Here's how the part is built. I have some questions about the finished solid (model axes, mm). Face numbers are marked on the shaded views. A direction names the side the tool comes from. Coordinates: 2 decimals unless noted, no trailing zeros. Loops run counter-clockwise (first coordinate to the right, second up) from the corner with the lowest first, then second, coordinate; pieces in that order, holes last.
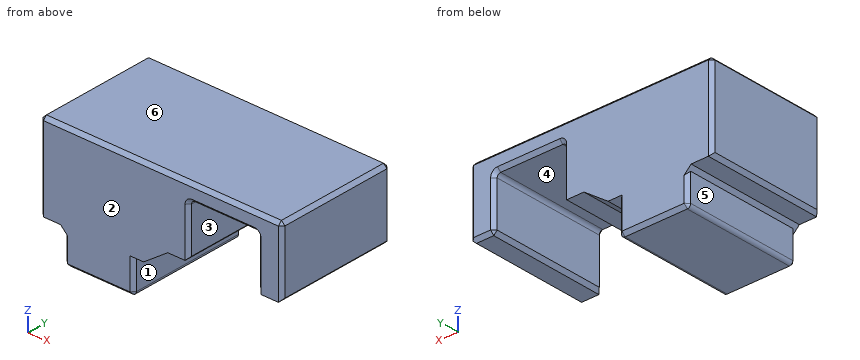
```python
from build123d import *

# Parameters (mm, degrees)
F1_DEPTH = 17.5
F2_SIZE  = 1
F3_R     = 1
F4_SIZE  = 1


with BuildPart() as f1:
    # F0 (on Front) → F1 (new body, symmetric)
    with BuildSketch(Plane.XZ):
        Polygon((33.969838, 0), (40.969838, 0), (40.969838, 20), (-29.030162, 20), (-29.030162, -5), (-22.030162, -5), (-22.030162, -15), (-2.030162, -15), (-2.030162, -5), (0.98608, -5), (7.969838, 0), (13.969838, 0), (13.969838, 15), (33.969838, 15), align=None)
    extrude(amount=F1_DEPTH, both=True)

    # F2
    f2_edges = [f1.edges().sort_by_distance(p)[0] for p in [
        (40.969838, 0, 0),
        (40.969838, -17.5, 10),
        (40.969838, 0, 20),
        (40.969838, 17.5, 10),
        (5.969838, -17.5, 20),
        (5.969838, 17.5, 20),
        (-29.030162, 0, 20),
        (-29.030162, -17.5, 7.5),
        (-29.030162, 17.5, 7.5),
        (-29.030162, 0, -5),
        (-22.030162, 0, -5),
    ]]
    chamfer(f2_edges, length=F2_SIZE)

    # F3
    f3_edges = [f1.edges().sort_by_distance(p)[0] for p in [
        (-22.030162, 0, -15),
        (-2.030162, 0, -15),
        (13.969838, 0, 15),
        (33.969838, 0, 15),
    ]]
    fillet(f3_edges, radius=F3_R)

    # F4
    f4_edges = [f1.edges().sort_by_distance(p)[0] for p in [
        (33.969838, 0, 0),
        (36.969838, 17.5, 0),
        (13.969838, 0, 0),
        (23.969838, -17.5, 15),
        (23.969838, 17.5, 15),
        (-12.030162, 17.5, -15),
        (-12.030162, -17.5, -15),
    ]]
    chamfer(f4_edges, length=F4_SIZE)


solid = f1.part
```
1. I want a section at A-A (z = 3.5). Please give me the cut outline in (x, y), then the cut area to 3 significant figures.
2. On a 3-axis mill with a long thin cutter (end or side, diameter ignored), from which of +Z, -Z, +X, -X, +Y, -Y can I reach the whole of each face in a straight line? I mean the marked faces 4, 5 and 6. Say none if no direction works.
3. I want a section at C-C (y = -1). Please give me the cut outline in (x, z), then the cut area to 3 significant figures.
4. We'd pull the mould along X, two halves only. Please class the marked faces 1, 2 and 3: +X half, -X half, draft (parallel to the pull), parting line (faces both ways), or undercut.
5. I want a section at B-B (x = 20). Please give me the cut outline in (y, z).
6. For pin 1 (12 mm diameter, centred on y = -7.5, z = -10, fed in from +X); pin 2 (2 mm diameter, centred on x = 32.5, y = -11, fed in from -Z); pin 3 (10 mm diameter, centred on y = 0.5, z = -10.5, fed in from +X), each with a flat end and sliding along its axis, tell me the tip position at first contact or that it passes through.
7. I want a section at D-D (z = -2). Please give me the cut outline in (x, y).
8. I need wall thicknesses on line 1 along X through (y, z) = (2, 7.5); line 2 along X through (y, z) = (15, -6.5); line 3 along Z through (x, y) = (10, -0.5). Which ranges of each line are inside material? Lowest first, please.
Response values:
1. outline: (-29.03, -16.5) - (-28.03, -17.5) - (12.97, -17.5) - (13.97, -16.5) - (13.97, 16.5) - (12.97, 17.5) - (-28.03, 17.5) - (-29.03, 16.5) - close; (33.97, -16.5) - (34.97, -17.5) - (39.97, -17.5) - (40.97, -16.5) - (40.97, 16.5) - (39.97, 17.5) - (34.97, 17.5) - (33.97, 16.5) - close
1. area: 1,750 mm2
2. face 4: -Z, +Y, -Y
2. face 5: -Z, -X, +Y, -Y
2. face 6: +Z, +X, -X, +Y, -Y
3. outline: (-29.03, -4) - (-28.03, -5) - (-23.03, -5) - (-22.03, -6) - (-22.03, -14) arc R1 ccw to (-21.03, -15) - (-3.03, -15) arc R1 ccw to (-2.03, -14) - (-2.03, -5) - (0.99, -5) - (7.97, 0) - (12.97, 0) - (13.97, 1) - (13.97, 14) arc R1 cw to (14.97, 15) - (32.97, 15) arc R1 cw to (33.97, 14) - (33.97, 1) - (34.97, 0) - (39.97, 0) - (40.97, 1) - (40.97, 19) - (39.97, 20) - (-28.03, 20) - (-29.03, 19) - close
3. area: 1,470 mm2
4. face 1: +X half
4. face 2: draft
4. face 3: undercut
5. outline: (-17.5, 16) - (-16.5, 15) - (16.5, 15) - (17.5, 16) - (17.5, 19) - (16.5, 20) - (-16.5, 20) - (-17.5, 19) - close
6. pin 1: stops at x = 2.38
6. pin 2: stops at z = 14.85
6. pin 3: stops at x = -2.03
7. outline: (-29.03, -16.5) - (-28.03, -17.5) - (5.18, -17.5) - (5.18, 17.5) - (-28.03, 17.5) - (-29.03, 16.5) - close
8. line 1: x = -29.03 to 13.97, 33.97 to 40.97
8. line 2: x = -22.03 to -2.03
8. line 3: z = 0 to 20
